Verification items for the finished model (mm, model axes). Face numbers are marked on the shaded views. A direction names the side the tool comes from. Coordinates: 2 decimals unless noted, no trailing zeros. Order: outer loops, then holes, each group sorted by start corner. A loop starts at its lowest first (then second) coordinate and runs counter-clockwise, first axis right, second up. Notation, with made-up numbers: M 28.25,3 L 44.25,3 A8 cw 44.25,14 Z; hole C -24.75,-11.5 d9. An arc over 180 degrees is marked long. Write item = value, one per line.
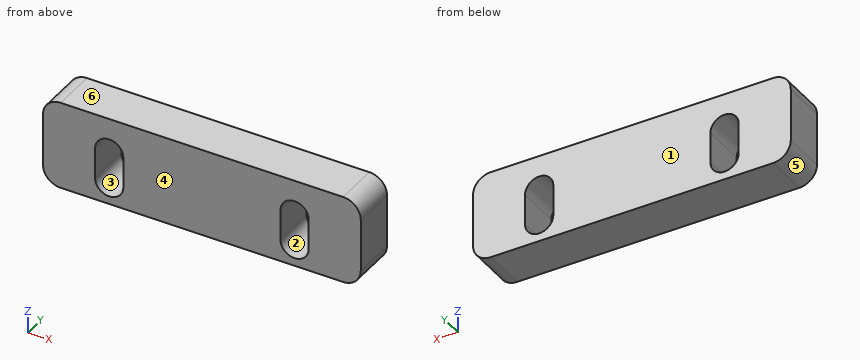
Autodesk Inventor part; units mm, degrees
ref_plane "YZ Plane" through (0, 0, 0) normal (1, 0, 0) x (0, 1, 0)
ref_plane "XZ Plane" through (0, 0, 0) normal (0, 1, 0) x (-1, 0, 0)
ref_plane "XY Plane" through (0, 0, 0) normal (0, 0, 1) x (1, 0, 0)
sketch "Sketch1" plane through (0, 0, 0) normal (0, 1, 0) x (-1, 0, 0)
  line L0 (0, 0) -> (36, 0)
  line L1 (36, 0) -> (36, -10)
  line L2 (36, -10) -> (0, -10)
  line L3 (0, -10) -> (0, 0)
  line L4 (18, 26.1157) -> (18, -38.8106) construction
  line L5 (28.5, 12.3286) -> (28.5, -24.6324) construction
  line L6 (7.5, 13.3064) -> (7.5, -23.3613) construction
  line L7 (28.5, -7.5) -> (28.5, -4) construction
  line L8 (30.1, -7.5) -> (30.1, -4)
  line L9 (26.9, -4) -> (26.9, -7.5)
  arc A0 (26.9, -7.5) -> (30.1, -7.5) centre (28.5, -7.5) ccw
  arc A1 (30.1, -4) -> (26.9, -4) centre (28.5, -4) ccw
  line L10 (7.5, -7.5) -> (7.5, -4) construction
  line L11 (5.9, -7.5) -> (5.9, -4)
  line L12 (9.1, -4) -> (9.1, -7.5)
  arc A2 (5.9, -7.5) -> (9.1, -7.5) centre (7.5, -7.5) ccw
  arc A3 (9.1, -4) -> (5.9, -4) centre (7.5, -4) ccw
  point P0 (18, 0)
  point P1 (28.5, -5.75)
  point P2 (7.5, -5.75)
  dimension "d0" = 36
  dimension "d1" = 10
  dimension "d2" = 21
  dimension "d3" = 3.5
  dimension "d4" = 3.2
  dimension "d5" = 2.5
extrude "Extrusion1" add sketch "Sketch1" along normal blind 5
fillet "Fillet1" radius 2 4 edges at (0, 2.5, 0) (0, 2.5, -10) (-36, 2.5, -10) (-36, 2.5, 0)
properties part number "LipoBat Spacer"
Item 1: Tool access check on the marked faces 1 and 2. Record the directions out of +Z, -Z, +X, -X, +Y, -Y that give a thin tool (end or side, any length) a straight path to the whole face; none if there is none.
Report:
face_1 = +Z, -Z, +X, -X, +Y
face_2 = +Y, -Y
Item 2: Sectioned sample at A-A, the plane y = 0.7. Enter the section's corners in (x, z), then the cut area to 3 significant figures.
Report:
outline = M -36,-8 A2 ccw -34,-10 L -2,-10 A2 ccw 0,-8 L 0,-2 A2 ccw -2,0 L -34,0 A2 ccw -36,-2 Z; hole M -30.1,-7.5 A1.6 ccw -26.9,-7.5 L -26.9,-4 A1.6 ccw -30.1,-4 Z; hole M -9.1,-7.5 A1.6 ccw -5.9,-7.5 L -5.9,-4 A1.6 ccw -9.1,-4 Z
area = 318 mm^2
Item 3: Sectioned sample at B-B, the plane z = -6. Enter the section's corners in (x, y).
Report:
outline = M -36,0 L -30.1,0 L -30.1,5 L -36,5 Z; M -26.9,0 L -9.1,0 L -9.1,5 L -26.9,5 Z; M -5.9,0 L 0,0 L 0,5 L -5.9,5 Z
Item 4: Release check for a two-part mould opening along Z. For the marked faces 3, 4, 5 and 6 record: pulls with the +Z half, pulls with the -Z half, needs draft (parallel to the pull), parting line crosses it, or undercut.
Report:
face_3 = undercut
face_4 = needs draft
face_5 = pulls with the -Z half
face_6 = pulls with the +Z half
Item 5: Scan lines: L1, parallel to X at y = 3.7, z = -5.5; L2, parallel to X at y = 1.75, z = -8.25; L3, parallel to Z at x = -28.5, y = 2.65. Record each from-to range of solid material in increasing order. Write a range as from..to.
Report:
L1 = -36..-30.1, -26.9..-9.1, -5.9..0
L2 = -35.98..-29.91, -27.09..-8.91, -6.09..-0.02
L3 = -10..-9.1, -2.4..0
Item 6: Sectioned sample at C-C, the plane x = -28.5. Enter the section's corners in (y, z), then the cut area to 3 significant figures.
Report:
outline = M 0,-10 L 5,-10 L 5,-9.1 L 0,-9.1 Z; M 0,-2.4 L 5,-2.4 L 5,0 L 0,0 Z
area = 16.5 mm^2
Item 7: Sectioned sample at D-D, the plane z = -8.75. Enter the section's corners in (x, y).
Report:
outline = M -35.85,0 L -29.5,0 L -29.5,5 L -35.85,5 Z; M -27.5,0 L -8.5,0 L -8.5,5 L -27.5,5 Z; M -6.5,0 L -0.15,0 L -0.15,5 L -6.5,5 Z
Item 8: Gauge pin test, flat end, axial feed: pin 1 (2 mm diameter, centred on x = -16.5, z = -4, fed in from -Y). Record the tip position at first contact, or that the pin passes through.
Report:
pin_1 = 0
